Here's the drawing with two shaded views (mm, measured from the low corner). I have some questions. Round coordinates to 2 decimals unless told otherwise and drop trailing zeros. Loops run counter-clockwise (first coordinate to the right, second up) from the corner with the lowest first, then second, coordinate; pieces in that order, holes last.
(1) If I drill on line 1 along Z through (x, y) = (140, 2.4); line 2 along X through (y, z) = (2.2, 80); line 3 along X through (y, z) = (1.7, 256.5), over which ranges is the centre line in solid material (lowest first)?
(2) Will these pins go through, and if not, where does the flat tip stop? pin 1 Ø10.5 at (x, z) = (243.92, 80) entering from +Y; pin 2 Ø6.5 at (x, z) = (140, 20) entering from -Y.
(3) I want a section at C-C on z = 260. Write out the boundary of the cut face in (x, y).
(4) I want a section at D-D on z = 200. Write out the boundary of the cut face in (x, y), plus the area to 3 significant figures.
(5) I want a section at B-B on y = 1.15. Write out the boundary of the cut face in (x, z).
(6) I want a section at A-A on x = 140. Write out the boundary of the cut face in (y, z), plus the area to 3 significant figures.
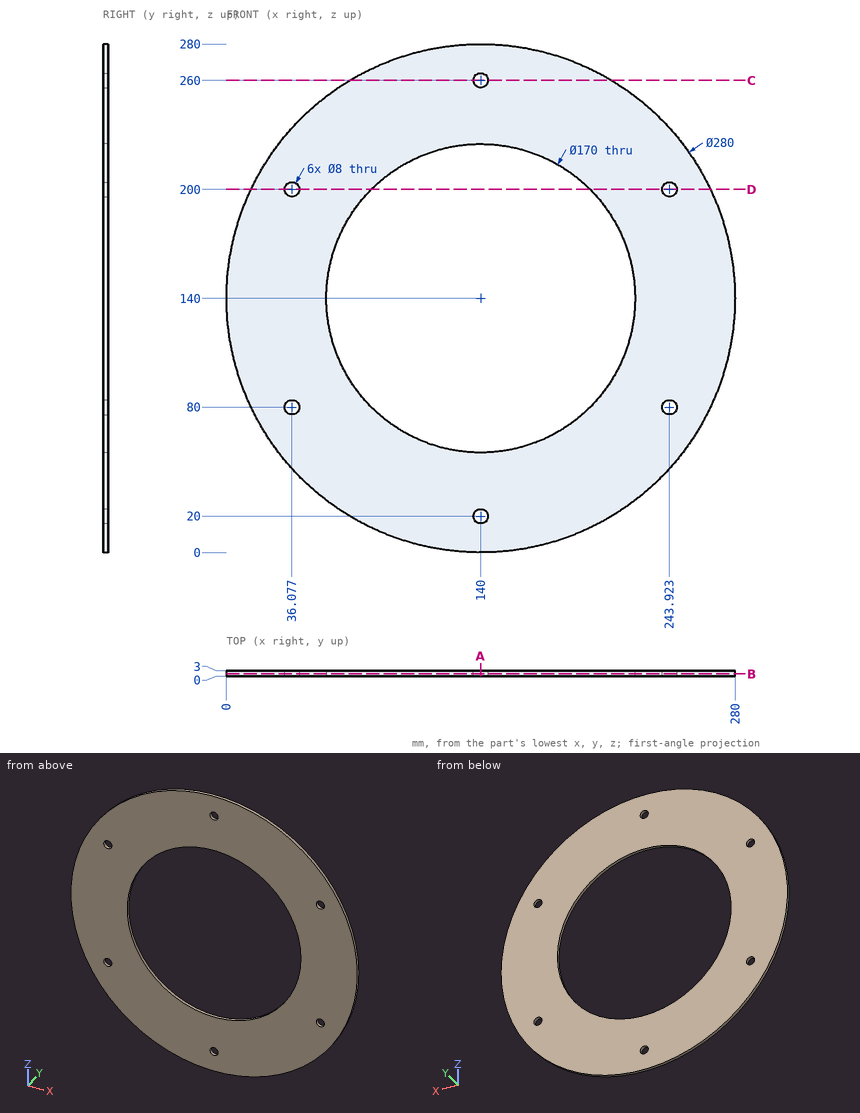
Filled sheet:
1. line 1: z = 0 to 16, 24 to 55, 225 to 256, 264 to 280
1. line 2: x = 13.51 to 32.08, 40.08 to 79.79, 200.21 to 239.92, 247.92 to 266.49
1. line 3: x = 62.36 to 138.06, 141.94 to 217.64
2. pin 1: stops at y = 3
2. pin 2: passes through
3. outline: (67.89, 0) - (136, 0) - (136, 3) - (67.89, 3) - close; (144, 0) - (212.11, 0) - (212.11, 3) - (144, 3) - close
4. outline: (13.51, 0) - (32.08, 0) - (32.08, 3) - (13.51, 3) - close; (40.08, 0) - (79.79, 0) - (79.79, 3) - (40.08, 3) - close; (200.21, 0) - (239.92, 0) - (239.92, 3) - (200.21, 3) - close; (247.92, 0) - (266.49, 0) - (266.49, 3) - (247.92, 3) - close
4. area: 350 mm2
5. outline: circle Ø280 at (140, 140); hole circle Ø8 at (36.08, 80); hole circle Ø8 at (36.08, 200); hole circle Ø170 at (140, 140); hole circle Ø8 at (140, 20); hole circle Ø8 at (140, 260); hole circle Ø8 at (243.92, 80); hole circle Ø8 at (243.92, 200)
6. outline: (0, 0) - (3, 0) - (3, 16) - (0, 16) - close; (0, 24) - (3, 24) - (3, 55) - (0, 55) - close; (0, 225) - (3, 225) - (3, 256) - (0, 256) - close; (0, 264) - (3, 264) - (3, 280) - (0, 280) - close
6. area: 282 mm2
